from build123d import *

# Parameters (mm, degrees)
F0_W       = 150.5549252033
F0_H       = 153.845757246
F1_DEPTH   = 40
F2_W       = 150.5549252033
F2_H       = 153.845757246
F3_DEPTH   = 40
F4_W       = 150.5549252033
F4_H       = 80
F4_R       = 2.7459354745
F3_FACE_W  = 150.5549252033
F3_FACE_H  = 80
F3_FACE1_W = 150.5549252033
F3_FACE1_H = 80
F5_DEPTH   = 40
F6_W       = 175.8493036032
F6_H       = 126.634541899
F7_DEPTH   = 40
F9_W       = 86.0539241694
F9_H       = 80.1538974047
F10_DEPTH  = 40
F11_W      = 113.8785094954
F11_H      = 80.3718343377
F12_DEPTH  = 40
F13_W      = 153.6099761724
F13_H      = 152.900993824
F14_DEPTH  = 40


with BuildPart() as f1:
    # F0 (on Top) → F1 (new body)
    with BuildSketch(Plane.XY):
        Rectangle(F0_W, F0_H)
    extrude(amount=F1_DEPTH)

    # F2 (on face) → F3 (join)
    with BuildSketch(Plane(origin=(0, 0, 0), x_dir=(1, 0, 0), z_dir=(0, 0, -1))):
        Rectangle(F2_W, F2_H)
    extrude(amount=F3_DEPTH)

    # F4 (on face) + F3_face (on face) + F3_face1 (on face) → F5 (join)
    with BuildSketch(Plane(origin=(0, 76.922878623, 0), x_dir=(-1, 0, 0), z_dir=(0, 1, 0))):
        Rectangle(F4_W, F4_H)
        Circle(F4_R, mode=Mode.SUBTRACT)
        Circle(F4_R)
    with BuildSketch(Plane(origin=(0, 76.922878623, 0), x_dir=(-1, 0, 0), z_dir=(0, 1, 0))):
        Rectangle(F3_FACE_W, F3_FACE_H)
    with BuildSketch(Plane.XZ.offset(76.922878623)):
        Rectangle(F3_FACE1_W, F3_FACE1_H)
    extrude(amount=F5_DEPTH, dir=(0, 1, 0))

    # F6 (on face) → F7 (join)
    with BuildSketch(Plane.XZ.offset(76.922878623)):
        with Locations((0, 8.4902700037)):
            Rectangle(F6_W, F6_H)
    extrude(amount=F7_DEPTH)

    # F9 (on face) → F10 (join)
    with BuildSketch(Plane.YZ.offset(75.2774626017)):
        with Locations((-38.1367646623, 40.0769487023)):
            Rectangle(F9_W, F9_H)
    extrude(amount=F10_DEPTH)

    # F11 (on face) → F12 (join)
    with BuildSketch(Plane.YZ.offset(75.2774626017)):
        with Locations((61.8294521701, 40.1859171689)):
            Rectangle(F11_W, F11_H)
    extrude(amount=F12_DEPTH)

    # F13 (on face) → F14 (join)
    with BuildSketch(Plane(origin=(0, 116.922878623, 0), x_dir=(-1, 0, 0), z_dir=(0, 1, 0))):
        Rectangle(F13_W, F13_H)
    extrude(amount=F14_DEPTH)


solid = f1.part
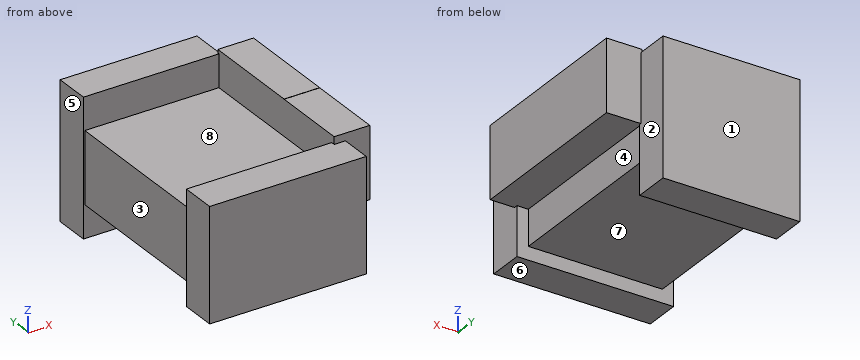
Verification items for the finished model (mm, model axes). Face numbers are marked on the shaded views. A direction names the side the tool comes from. Give positions to 0.01 mm unless a question says otherwise; leave off trailing zeros. Loops run counter-clockwise (first coordinate to the right, second up) from the corner with the lowest first, then second, coordinate; pieces in that order, holes last.
1) Sectioned sample at D-D, the plane z = 3.5. Enter the section's corners in (x, y).
2) Draft check along Y on the marked faces 1, 2 and 3. Enter one of: pulls with the +Y half, pulls with the -Y half, needs draft (parallel to the pull), parting line crosses it, or undercut.
3) Depth check by flat-ended pin: pin 1 Ø20 at (y, z) = (145.5, -1) entering from +X (3 decimals); pin 2 Ø12 at (y, z) = (-10, 62) entering from -X; pin 3 Ø12 at (x, y) = (19, 135) entering from +Z. Enter the tip coordinate at first touch or a pass-through.
4) Sectioned sample at A-A, the plane z = -48.5. Enter the section's corners in (x, y).
5) Sectioned sample at B-B, the plane y = 21.5. Enter the section's corners in (x, z).
6) Set-up check for the marked faces 4, 5, 6, 7 and 8: record each of +Z, -Z, +X, -X, +Y, -Y from which the full face is reachable in a straight line by a thin tool's end or side.
7) Thickness scan on line 1 along Y through (x, z) = (-13, 56); line 2 along Y through (x, z) = (-48, -61); line 3 along Z through (x, y) = (32, -48). Record the ranges inside material, lowest first.
8) Sectioned sample at C-C, the plane x = 36.5. Enter the section's corners in (y, z).
Answers:
1. outline: (-87.92, -116.92) - (87.92, -116.92) - (87.92, -81.16) - (115.28, -81.16) - (115.28, 118.77) - (76.8, 118.77) - (76.8, 156.92) - (-76.8, 156.92) - (-76.8, 116.92) - (-75.28, 116.92) - (-75.28, -76.92) - (-87.92, -76.92) - close
2. face 1: pulls with the +Y half
2. face 2: needs draft
2. face 3: undercut
3. pin 1: stops at x = 76.805
3. pin 2: stops at x = 75.28
3. pin 3: stops at z = 76.45
4. outline: (-87.92, -116.92) - (87.92, -116.92) - (87.92, -76.92) - (-87.92, -76.92) - close; (-76.8, 116.92) - (76.8, 116.92) - (76.8, 156.92) - (-76.8, 156.92) - close
5. outline: (-75.28, -40) - (75.28, -40) - (75.28, 0) - (115.28, 0) - (115.28, 80.37) - (75.28, 80.37) - (75.28, 40) - (-75.28, 40) - close
6. face 4: -Z, +X
6. face 5: +Z, -Z, -X, +Y
6. face 6: -Z, +X, -X, -Y
6. face 7: -Z, +X, -X
6. face 8: +Z, -X
7. line 1: y = -116.92 to -76.92, 116.92 to 156.92
7. line 2: y = 116.92 to 156.92
7. line 3: z = -40 to 40
8. outline: (-116.92, -54.83) - (-76.92, -54.83) - (-76.92, -40) - (116.92, -40) - (116.92, -76.45) - (156.92, -76.45) - (156.92, 76.45) - (116.92, 76.45) - (116.92, 40) - (-76.92, 40) - (-76.92, 71.81) - (-116.92, 71.81) - close
